```python
from build123d import *

# Parameters (mm, degrees)
SKETCH1_R              = 1.55
EXTRUDE_707_DEPTH      = 2.4
SKETCH2_W              = 31
SKETCH2_H              = 31
SKETCH2_W_2            = 26
SKETCH2_H_2            = 26
GPS_DEPTH              = 9.5
GPS_2_R                = 1.75
CHAMFER_1832_SIZE      = 1
EXTRUDE_3171_DEPTH     = 6.5
SKETCH4_R              = 2.125
CUT_EXTRUDE_3634_DEPTH = 73.664551053
CUT_EXTRUDE_3926_DEPTH = 65.212061635
SKETCH7_W              = 14
SKETCH7_H              = 6.75
SKETCH7_W_2            = 14.827228548
CUT_EXTRUDE_4854_DEPTH = 6.5
SKETCH8_W              = 4
SKETCH8_H              = 17.5
CUT_EXTRUDE_5206_DEPTH = 0.5
CHAMFER_5287_SIZE      = 1
SKETCH9_W              = 8
SKETCH9_H              = 77.991423638
CUT_EXTRUDE_6206_DEPTH = 0.5


with BuildPart() as part:
    # Sketch1 → Extrude 707 (new body)
    with BuildSketch(Plane(origin=(0, 0, 0), x_dir=(1, 0, 0), z_dir=(0, 1, 0))):
        with BuildLine():
            Line((-26.041067799, 38.995711819), (26.041067799, 38.995711819))
            Line((26.041067799, 38.995711819), (26.041067799, 28.995711819))
            Line((26.041067799, 28.995711819), (30.074330581, 28.995711819))
            ThreePointArc((30.074330581, 28.995711819), (34.107558501, 24.94567978), (30.040792356, 20.929325701))
            Line((30.040792356, 20.929325701), (26.041067799, 20.929325701))
            Line((26.041067799, 20.929325701), (26.041067799, -11.037902063))
            Line((26.041067799, -11.037902063), (30.074330581, -11.037902063))
            ThreePointArc((30.074330581, -11.037902063), (34.107558501, -15.087934101), (30.040792356, -19.104288181))
            Line((30.040792356, -19.104288181), (26.041067799, -19.104288181))
            Line((26.041067799, -19.104288181), (26.041067799, -32.550614881))
            Line((26.041067799, -32.550614881), (22.539090807, -38.995711819))
            Line((22.539090807, -38.995711819), (-22.539090807, -38.995711819))
            Line((-22.539090807, -38.995711819), (-26.041067799, -32.550614881))
            Line((-26.041067799, -32.550614881), (-26.041067799, -19.104288181))
            Line((-26.041067799, -19.104288181), (-30.040792356, -19.104288181))
            ThreePointArc((-30.040792356, -19.104288181), (-34.107558501, -15.087934101), (-30.074330581, -11.037902063))
            Line((-30.074330581, -11.037902063), (-26.041067799, -11.037902063))
            Line((-26.041067799, -11.037902063), (-26.041067799, 20.929325701))
            Line((-26.041067799, 20.929325701), (-30.040792356, 20.929325701))
            ThreePointArc((-30.040792356, 20.929325701), (-34.107558501, 24.94567978), (-30.074330581, 28.995711819))
            Line((-30.074330581, 28.995711819), (-26.041067799, 28.995711819))
            Line((-26.041067799, 28.995711819), (-26.041067799, 38.995711819))
        make_face()
        with Locations(Location((-30.041067799, 24.962449038, 0), (0, 0, 270))):
            Circle(SKETCH1_R, mode=Mode.SUBTRACT)
        with Locations(Location((30.041067799, 24.962449038, 0), (0, 0, 90))):
            Circle(SKETCH1_R, mode=Mode.SUBTRACT)
        with Locations(Location((-30.041067799, -15.071164844, 0), (0, 0, 270))):
            Circle(SKETCH1_R, mode=Mode.SUBTRACT)
        with Locations(Location((30.041067799, -15.071164844, 0), (0, 0, 90))):
            Circle(SKETCH1_R, mode=Mode.SUBTRACT)
    extrude(amount=EXTRUDE_707_DEPTH)

    # Sketch2 → GPS (add)
    with BuildSketch(Plane(origin=(0, 2.4, 0), x_dir=(1, 0, 0), z_dir=(0, 1, 0))):
        Rectangle(SKETCH2_W, SKETCH2_H)
        Rectangle(SKETCH2_W_2, SKETCH2_H_2, mode=Mode.SUBTRACT)
    extrude(amount=GPS_DEPTH)

    # GPS 2
    gps_2_edges = [part.edges().sort_by_distance(p)[0] for p in [
        (15.5, 7.15, -15.5),
        (-15.5, 7.15, -15.5),
        (-15.5, 7.15, 15.5),
        (15.5, 7.15, 15.5),
    ]]
    fillet(gps_2_edges, radius=GPS_2_R)

    # Chamfer 1832
    chamfer_1832_edges = [part.edges().sort_by_distance(p)[0] for p in [
        (-30.041067799, 2.4, -26.512449038),
        (30.041067799, 2.4, -23.412449038),
        (30.041067799, 2.4, 16.621164844),
        (-30.041067799, 2.4, 13.521164844),
    ]]
    chamfer(chamfer_1832_edges, length=CHAMFER_1832_SIZE)

    # Sketch3 → Extrude 3171 (add)
    with BuildSketch(Plane(origin=(0, 2.4, 0), x_dir=(1, 0, 0), z_dir=(0, 1, 0))):
        Polygon((-24.467823985, -16.04483058), (-15.5, -7.229070577), (-15.5, -4.529331749), (-26.041067799, -15.596764458), (-26.041067799, -23.659714375), (-20.467823985, -23.659714375), (-7.413614274, -15.5), (-9.413614274, -15.5), (-20.467823985, -21.659714375), align=None)
        Polygon((9.413614274, -15.5), (7.413614274, -15.5), (20.467823985, -23.659714375), (26.041067799, -23.659714375), (26.041067799, -15.596764458), (15.5, -4.529331749), (15.5, -7.229070577), (24.467823985, -16.04483058), (20.467823985, -21.659714375), align=None)
    extrude(amount=EXTRUDE_3171_DEPTH)

    # Sketch4 → Cut-Extrude 3634 (cut, through all)
    with BuildSketch(Plane.ZY.offset(26.041067799)):
        with Locations((19.852272478, 5.65)):
            Circle(SKETCH4_R)
    extrude(amount=-CUT_EXTRUDE_3634_DEPTH, mode=Mode.SUBTRACT)

    # Sketch6 → Cut-Extrude 3926 (cut, through all)
    with BuildSketch(Plane.ZY.offset(15.5)):
        with BuildLine():
            Line((-9, 9.4), (-0.220668251, 9.4))
            ThreePointArc((-0.220668251, 9.4), (2.029331749, 7.15), (-0.220668251, 4.9))
            Line((-0.220668251, 4.9), (-9, 4.9))
            ThreePointArc((-9, 4.9), (-11.25, 7.15), (-9, 9.4))
        make_face()
    extrude(amount=-CUT_EXTRUDE_3926_DEPTH, mode=Mode.SUBTRACT)

    # Sketch7 → Cut-Extrude 4854 (cut)
    with BuildSketch(Plane(origin=(0, 0, 0), x_dir=(1, 0, 0), z_dir=(0, 1, 0))):
        with Locations((0, 12.125)):
            Rectangle(SKETCH7_W, SKETCH7_H)
        with Locations((0, -12.125)):
            Rectangle(SKETCH7_W_2, SKETCH7_H)
    extrude(amount=CUT_EXTRUDE_4854_DEPTH, mode=Mode.SUBTRACT)

    # Sketch8 → Cut-Extrude 5206 (cut)
    with BuildSketch(Plane(origin=(0, 2.4, 0), x_dir=(1, 0, 0), z_dir=(0, 1, 0))):
        Rectangle(SKETCH8_W, SKETCH8_H)
    extrude(amount=-CUT_EXTRUDE_5206_DEPTH, mode=Mode.SUBTRACT)

    # Chamfer 5287
    chamfer_5287_edges = [part.edges().sort_by_distance(p)[0] for p in [
        (4.5, 2.4, -8.75),
        (0, 2.4, -15.5),
        (-4.706807137, 2.4, 8.75),
    ]]
    chamfer(chamfer_5287_edges, length=CHAMFER_5287_SIZE)

    # Sketch9 → Cut-Extrude 6206 (cut)
    with BuildSketch(Plane.XZ):
        Rectangle(SKETCH9_W, SKETCH9_H)
    extrude(amount=-CUT_EXTRUDE_6206_DEPTH, mode=Mode.SUBTRACT)


solid = part.part
```
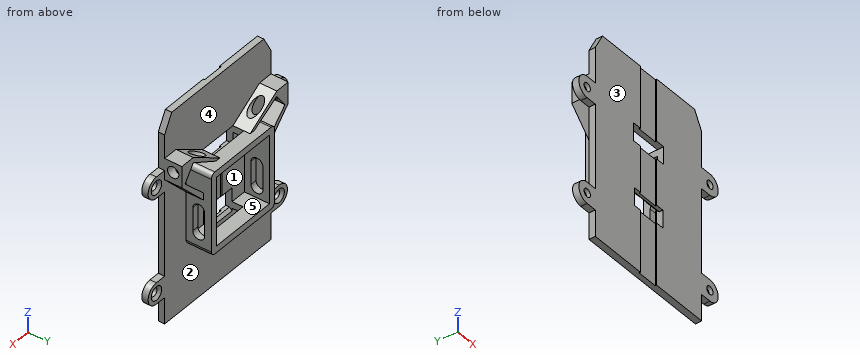
The model under review builds one solid part; all positions refer to its coordinate system, in mm. Face numbers are marked on the shaded views. A direction names the side the tool comes from. Round coordinates to 2 decimals unless told otherwise and drop trailing zeros. Order: outer loops, then holes, each group sorted by start corner. A loop starts at its lowest first (then second) coordinate and runs counter-clockwise, first axis right, second up.
Item 1: Add section B-B, the plane x = -5. State the section outline as (y, z) points.
Working result:
outline: (0, -39) - (2.4, -39) - (2.4, -16.5) - (1.4, -15.5) - (0, -15.5) - close; (0, -8.75) - (1.4, -8.75) - (2.4, -7.75) - (2.4, 7.75) - (1.4, 8.75) - (0, 8.75) - close; (0, 15.5) - (2.4, 15.5) - (2.4, 39) - (0, 39) - close; (6.5, -15.5) - (11.9, -15.5) - (11.9, -13) - (6.5, -13) - close; (6.5, 13) - (11.9, 13) - (11.9, 15.5) - (6.5, 15.5) - close
Item 2: Machinability: for the marked faces 3, 4 and 5, which of the approach directions +Z, -Z, +X, -X, +Y, -Y give a long, thin tool a straight path to every point of the face, cutting with its end or side? Answer none if there is none.
Working result:
face 3: +Z, -Z, +X, -X, -Y
face 4: +Z, +Y
face 5: +Y
Item 3: To check wall thickness, follow probe 1 along X at (y, z) = (9.5, -4); probe 2 along X at (y, z) = (7.75, 8); probe 3 along X at (y, z) = (6, 17). State the ranges of each line that lie inside material, in increasing order.
Working result:
probe 1: x = -15.5 to -13, 13 to 15.5
probe 2: x = -18.81 to -16.28, -15.5 to -13, 13 to 15.5, 16.28 to 18.81
probe 3: x = -26.04 to -23.79, -12.11 to -9.81, 9.81 to 12.11, 23.79 to 26.04
Item 4: For pin 1 (2.5 mm diameter, centred on x = -29, y = 0.5, fed in from +Z); pin 2 (1.5 mm diameter, centred on x = 15, y = 6.5, fed in from -Z); pin 3 (1.2 mm diameter, centred on y = 1, z = -34.5, fed in from +X), all flat-tipped, find the tip position at first contact; note any pin that passes through.
Working result:
pin 1: stops at z = 19.1
pin 2: stops at z = -15.43
pin 3: stops at x = 26.04
Item 5: Add section A-A, the plane y = 10.75. State the section outline as (x, z) points, and give its area (3 significant figures).
Working result:
outline: (-15.5, -13.75) arc R1.75 ccw to (-13.75, -15.5) - (13.75, -15.5) arc R1.75 ccw to (15.5, -13.75) - (15.5, 13.75) arc R1.75 ccw to (13.75, 15.5) - (-13.75, 15.5) arc R1.75 ccw to (-15.5, 13.75) - close; hole (-13, -13) - (13, -13) - (13, 13) - (-13, 13) - close
area: 282 mm2
Item 6: Draft analysis for pull direction X (two halves, no side actions). For the marked faces 1 and 2, state which applies: released by +X, released by -X, zero draft, split by the parting line, or undercut.
Working result:
face 1: undercut
face 2: zero draft
